Autodesk Inventor part; units mm, degrees
ref_plane "YZ Plane" through (0, 0, 0) normal (1, 0, 0) x (0, 1, 0)
ref_plane "XZ Plane" through (0, 0, 0) normal (0, 1, 0) x (-1, 0, 0)
ref_plane "XY Plane" through (0, 0, 0) normal (0, 0, 1) x (1, 0, 0)
sketch "Sketch1" plane through (0, 0, 0) normal (0, 1, 0) x (-1, 0, 0)
  line L0 (0, 0) -> (350, 0)
  line L1 (350, 0) -> (350, -120)
  line L2 (350, -120) -> (0, -120)
  line L3 (0, -120) -> (0, 0)
  circle A0 centre (175, -31) radius 3.75
  circle A1 centre (245, -31) radius 3.75
  circle A2 centre (105, -28.4204) radius 3.75
  dimension "d0" = 350
  dimension "d1" = 120
  dimension "d2" = 7.5
  dimension "d3" = 31
  dimension "d4" = 7.5
  dimension "d5" = 7.5
  dimension "d6" = 70
  dimension "d7" = 70
extrude "Extrusion1" add sketch "Sketch1" along normal blind 6.35
sketch "Sketch2" plane through (0, 6.35, 0) normal (0, 1, 0) x (1, 0, 0)
  line L0 (0, 120) -> (-350, 120)
  line L1 (-192.5, 120) -> (-157.5, 120)
  line L2 (-157.5, 120) -> (-157.5, 80)
  line L3 (-157.5, 80) -> (-192.5, 80)
  line L4 (-192.5, 80) -> (-192.5, 120)
  line L5 (0, 0) -> (0, 120)
  dimension "d10" = 35
  dimension "d11" = 40
  dimension "d12" = 157.5
extrude "Extrusion2" add sketch "Sketch2" along normal blind 62
sketch "Sketch3" plane through (0, 68.35, 0) normal (0, 1, 0) x (1, 0, 0)
  circle A0 centre (-175, 114) radius 2.125
  line L0 (-157.5, 120) -> (-192.5, 120)
  circle A1 centre (-169, 114) radius 2.125
  circle A2 centre (-181, 114) radius 2.125
  point P0 (0, 0)
  dimension "d15" = 4.25
  dimension "d16" = 6
  dimension "d17" = 4.25
  dimension "d18" = 6
  dimension "d19" = 4.25
  dimension "d20" = 6
hole "Hole1" at (-181, 68.35, -114) at (-175, 68.35, -114) at (-169, 68.35, -114) direction (0, -1, 0) diameter 4.25 depth 8 tip angle 118
sketch "Sketch4" plane through (-192.5, 6.35, -120) normal (-1, 0, 0) x (0, 0, 1)
  point P0 (120, -6.35)
sketch "Sketch5" plane through (-192.5, 6.35, -120) normal (-1, 0, 0) x (0, 0, 1)
  line L0 (0, 0) -> (0, 62)
  line L1 (0, 42) -> (40, 42)
  line L2 (40, 0) -> (40, 62)
  line L3 (0, 62) -> (40, 62)
  circle A0 centre (6, 48) radius 1.5
  circle A1 centre (34, 48) radius 1.5
  point P0 (120, -6.35)
  dimension "d28" = 20
  dimension "d29" = 3
  dimension "d30" = 3
  dimension "d31" = 6
  dimension "d32" = 6
  dimension "d33" = 6
  dimension "d34" = 6
hole "Hole2" at (-192.5, 54.35, -86) at (-192.5, 54.35, -114) direction (1, 0, 0) diameter 3 depth 2 tip angle 118
sketch "Sketch6" plane through (-192.5, 6.35, -80) normal (0, 0, 1) x (1, 0, 0)
  line L0 (0, 42) -> (35, 42)
  line L1 (0, 62) -> (35, 62)
  circle A0 centre (6, 48) radius 1.5
  line L2 (0, 0) -> (0, 62)
  circle A1 centre (29, 48) radius 1.5
  line L3 (35, 0) -> (35, 62)
  point P0 (192.5, -6.35)
  dimension "d42" = 20
  dimension "d43" = 3
  dimension "d44" = 6
  dimension "d45" = 6
  dimension "d46" = 3
  dimension "d47" = 6
  dimension "d48" = 6
hole "Hole3" at (-186.5, 54.35, -80) at (-163.5, 54.35, -80) direction (0, 0, -1) diameter 3 depth 2 tip angle 118
sketch "Sketch7" plane through (-157.5, 6.35, -80) normal (1, 0, 0) x (0, 0, -1)
  circle A0 centre (6, 48) radius 1.5
  circle A1 centre (6, 48) radius 1.5
  circle A2 centre (34, 48) radius 1.5
  circle A3 centre (34, 48) radius 1.5
  point P0 (-80, -6.35)
  dimension "d56" = 3
  dimension "d57" = 3
hole "Hole4" at (-157.5, 54.35, -86) at (-157.5, 54.35, -114) direction (-1, 0, 0) diameter 3 depth 2 tip angle 118
properties part number "Base" material "Wood (Birch)"
Geometry: final body of the model. Coordinates: model frame, mm. A direction names the side the tool comes from. Coordinates: 2 decimals unless noted, no trailing zeros. Write each loop counter-clockwise with the first axis right and the second up, starting at its lowest first coordinate (ties: lowest second). Pieces come first, ordered by that corner, then holes. Notation, with made-up numbers: M 33,84 L 46,84 A27 ccw 46,113 Z; hole C 45.25,-31.5 d5. An arc over 180 degrees is marked long. Use CSV: the item, a comma, the result in double quotes. Start each with the question number.
1. Cut plane A-A on y = 23. Return the cut outline in (x, z), plus the area to 3 significant figures.
2. Ray query, probe 1 along Z at (x, y) = (-190.95, 54.35); probe 2 along X at (y, z) = (62, -114) (3 decimals); probe 3 along X at (y, z) = (54.35, -80.6). Return the intervals inside material, ascending.
3. Reachability of faces 1 (the face through (-172.236, 3.131, -33.534)), 2 (the face through (-192.5, 37, -100)) from +Z, -Z, +X, -X, +Y, -Y: full face, straight path, thin tool, end or side. Return the list, or none.
4. Mould query, pull axis X, two halves, no side actions, for faces 3 (the face through (-175, 37, -80)), 4 (the face through (-350, 3, -59)), 5 (the face through (-108.464, 3.131, -26.984)), 6 (the face through (-157.5, 37, -100)). Classes: pulls with the +X half, pulls with the -X half, needs draft (parallel to the pull), parting line crosses it, or undercut.
5. First-contact query: P1, Ø2, axis at x = -258.5, z = -27.5, coming from the -Y side; P2, Ø4, axis at y = 54.35, z = -114, coming from the -X side; P3, Ø10.5, axis at x = -169, y = 26.5, coming from the +Z side; P4, Ø4.5, axis at x = -175, z = -31, coming from the +Y side. Flat tips, straight axial feed; report the tip coordinate or a pass-through.
6. Cut plane B-B on z = -48. Return the cut outline in (x, y).
Entries:
1,outline,"M -192.5,-120 L -157.5,-120 L -157.5,-80 L -192.5,-80 Z"
1,area,"1,400 mm²"
2,probe 1,"-120 to -115.5, -112.5 to -87.5, -84.5 to -80"
2,probe 2,"-192.5 to -183.125, -178.875 to -177.125, -172.875 to -171.125, -166.875 to -157.5"
2,probe 3,"-192.5 to -188, -185 to -165, -162 to -157.5"
3,face 1,"+Y, -Y"
3,face 2,"+Z, -Z, -X, +Y"
4,face 3,"needs draft"
4,face 4,"pulls with the -X half"
4,face 5,"undercut"
4,face 6,"pulls with the +X half"
5,P1,"y = 0"
5,P2,"x = -192.5"
5,P3,"z = -80"
5,P4,"through"
6,outline,"M -350,0 L 0,0 L 0,6.35 L -350,6.35 Z"
